Read the model definition and answer for the solid it produces. Units are mm, in the model's axes. A direction names the side the tool comes from. Give positions to 0.01 mm unless a question says otherwise; leave off trailing zeros. Write each loop counter-clockwise with the first axis right and the second up, starting at its lowest first coordinate (ties: lowest second). Pieces come first, ordered by that corner, then holes.
```python
from build123d import *

# Parameters (mm, degrees)
BOSS_EXTRUDE1_DEPTH = 304.8
SHELL1_T            = -2.54
SKETCH4_W           = 50.8
SKETCH4_H           = 50.8
BOSS_EXTRUDE2_DEPTH = 381
SKETCH5_W           = 30.48
SKETCH5_H           = 279.4
CUT_EXTRUDE1_DEPTH  = 7.62
SKETCH6_W           = 63.5
SKETCH6_H           = 63.5
BOSS_EXTRUDE3_DEPTH = 2.54
SKETCH7_W           = 5.08
SKETCH7_H           = 63.5
BOSS_EXTRUDE4_DEPTH = 50.8
BOSS_EXTRUDE5_REACH = 1036.867
SKETCH8_R           = 19.05


with BuildPart() as part:
    # Sketch3 → Boss-Extrude1 (new body)
    with BuildSketch(Plane.XY):
        Polygon((427.867059624, 0), (352.824484244, 0), (352.824484244, 419.782362276), (121.685060077, 419.782362276), (121.685060077, 0), (46.642484697, 0), (46.642484697, 914.4), (121.685060077, 914.4), (121.685060077, 527.57832691), (352.824484244, 527.57832691), (352.824484244, 914.4), (427.867059624, 914.4), align=None)
    extrude(amount=-BOSS_EXTRUDE1_DEPTH)

    # Shell1
    shell1_openings = [part.faces().sort_by_distance(p)[0] for p in [
        (237.254772161, 459.732303747, -304.8),
    ]]
    offset(amount=SHELL1_T, openings=shell1_openings, kind=Kind.INTERSECTION)

    # Sketch4 → Boss-Extrude2 (add)
    with BuildSketch(Plane(origin=(0, 0, -2.54), x_dir=(-1, 0, 0), z_dir=(0, 0, -1))):
        with Locations((-237.254772161, 473.630362276)):
            Rectangle(SKETCH4_W, SKETCH4_H)
    extrude(amount=BOSS_EXTRUDE2_DEPTH)

    # Sketch5 → Cut-Extrude1 (cut)
    with BuildSketch(Plane.XZ.offset(-419.782362276)):
        with Locations((239.682484697, -165.1)):
            Rectangle(SKETCH5_W, SKETCH5_H)
    extrude(amount=-CUT_EXTRUDE1_DEPTH, mode=Mode.SUBTRACT)

    # Sketch6 → Boss-Extrude3 (add)
    with BuildSketch(Plane(origin=(0, 0, -383.54), x_dir=(-1, 0, 0), z_dir=(0, 0, -1))):
        with Locations((-237.254772161, 473.630362276)):
            Rectangle(SKETCH6_W, SKETCH6_H)
    extrude(amount=BOSS_EXTRUDE3_DEPTH)

    # Sketch7 → Boss-Extrude4 (add)
    with BuildSketch(Plane(origin=(0, 0, -386.08), x_dir=(-1, 0, 0), z_dir=(0, 0, -1))):
        with Locations((-258.844772161, 473.630362276)):
            Rectangle(SKETCH7_W, SKETCH7_H)
        with Locations((-215.664772161, 473.630362276)):
            Rectangle(SKETCH7_W, SKETCH7_H)
    extrude(amount=BOSS_EXTRUDE4_DEPTH)

    # Sketch8 → Boss-Extrude5 (add, up to next)
    with BuildSketch(Plane.ZY.offset(-256.304772161), mode=Mode.PRIVATE) as boss_extrude5_sk1:
        with Locations(Location((-411.48, 473.630362276, 0), (0, 0, 180))):
            Circle(SKETCH8_R)
    boss_extrude5_tool1 = extrude(boss_extrude5_sk1.sketch, amount=BOSS_EXTRUDE5_REACH, mode=Mode.PRIVATE) - part.part
    add(boss_extrude5_tool1.solids().sort_by_distance((256.304772, 473.630362, -411.48))[0])


solid = part.part
```
Item 1: Section C-C (x = 328.5) is taken. Write down the section's boundary in (y, z).
Result set:
outline: (419.78, -304.8) - (422.32, -304.8) - (422.32, -2.54) - (525.04, -2.54) - (525.04, -304.8) - (527.58, -304.8) - (527.58, 0) - (419.78, 0) - close
Item 2: Find the intervals of material crossed by line 1 along X through (y, z) = (691.5, -235); line 2 along Y through (x, z) = (204, -169.5); line 3 along Y through (x, z) = (102.5, -123.5), in increasing order.
Result set:
line 1: x = 46.64 to 49.18, 119.15 to 121.69, 352.82 to 355.36, 425.33 to 427.87
line 2: y = 419.78 to 422.32, 525.04 to 527.58
line 3: y = 0 to 2.54, 911.86 to 914.4
Item 3: Section A-A (z = -411.48) is taken. Write down the section's boundary in (x, y), and give its area (3 significant figures).
Result set:
outline: (213.12, 441.88) - (218.2, 441.88) - (218.2, 454.58) - (256.3, 454.58) - (256.3, 441.88) - (261.38, 441.88) - (261.38, 505.38) - (256.3, 505.38) - (256.3, 492.68) - (218.2, 492.68) - (218.2, 505.38) - (213.12, 505.38) - close
area: 2,100 mm2
Item 4: Section B-B (y = 762) is taken. Write down the section's boundary in (x, z).
Result set:
outline: (46.64, -304.8) - (49.18, -304.8) - (49.18, -2.54) - (119.15, -2.54) - (119.15, -304.8) - (121.69, -304.8) - (121.69, 0) - (46.64, 0) - close; (352.82, -304.8) - (355.36, -304.8) - (355.36, -2.54) - (425.33, -2.54) - (425.33, -304.8) - (427.87, -304.8) - (427.87, 0) - (352.82, 0) - close
Item 5: Each of these flat-tipped pins is pushed along its axis until it touches: pin 1 Ø2 at (x, z) = (290, -242.5) entering from -Y; pin 2 Ø2 at (y, z) = (463, -384.5) entering from +X; pin 3 Ø3 at (x, y) = (269.5, 504.5) entering from -Z. Where does it stop, or does it pass through?
Result set:
pin 1: stops at y = 419.78
pin 2: stops at x = 269
pin 3: stops at z = -386.08
Item 6: Section D-D (x = 371.5) is taken. Write down the section's boundary in (y, z), and give its area (3 significant figures).
Result set:
outline: (0, -304.8) - (2.54, -304.8) - (2.54, -2.54) - (911.86, -2.54) - (911.86, -304.8) - (914.4, -304.8) - (914.4, 0) - (0, 0) - close
area: 3,860 mm2
Item 7: Determine the mould class of faces 1 (the flat face through (121.685, 724, -150)), 2 (the flat face through (240, 464, 0)) for opening direction X: pulls with the +X half, pulls with the -X half, needs draft (parallel to the pull), parting line crosses it, or undercut.
Result set:
face 1: undercut
face 2: needs draft
Item 8: Which of the six approach directions +Z, -Z, +X, -X, +Y, -Y give full straight-line access (tool end or side, diameter ignored) to faces 3 (the flat face through (352.824, 207, -150)), 4 (the flat face through (49.182, 451, -152)), 5 (the flat face through (238, 448.23, -190)), 6 (the flat face through (391, 0, -150)), 7 (the flat face through (352.824, 718, -150))?
Result set:
face 3: +Z, -Z, -Y
face 4: -Z
face 5: none
face 6: +Z, -Z, +X, -X, -Y
face 7: +Z, -Z, +Y
